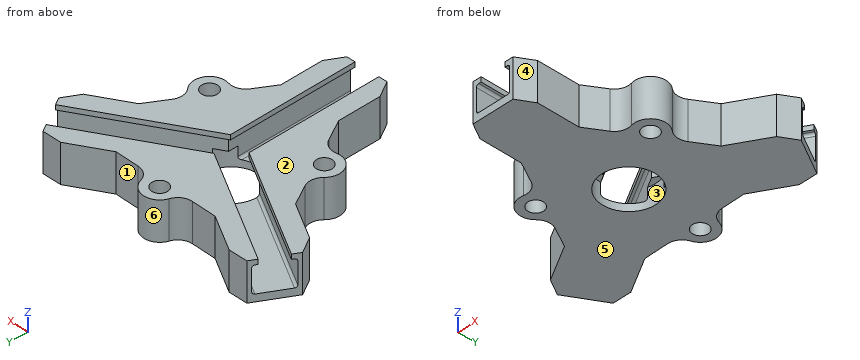
```python
from build123d import *

# Parameters (mm, degrees)
SKETCH1_R                        = 1.65
SKETCH1_R_2                      = 2.565
BOSS_EXTRUDE2_DEPTH              = 8
CUT_EXTRUDE1_REACH               = 80.832
CUT_EXTRUDE1_OFFSET_FROM_SURFACE = 13
CUT_EXTRUDE2_REACH               = 61.944
CUT_EXTRUDE2_OFFSET_FROM_SURFACE = 13
CUT_EXTRUDE3_REACH               = 80.174
CUT_EXTRUDE3_OFFSET_FROM_SURFACE = 13
FILLET1_R                        = 3
FILLET2_R                        = 0.5
SKETCH5_R                        = 5.6
CUT_EXTRUDE4_DEPTH               = 4


with BuildPart() as part:
    # Sketch1 → Boss-Extrude2 (new body)
    with BuildSketch(Plane.XY):
        with BuildLine():
            Line((-15.818539514, 20.899253914), (-23.777051469, 20.899253914))
            Line((-23.777051469, 20.899253914), (-31.392628778, 25.071578724))
            Line((-31.392628778, 25.071578724), (-35.221090626, 24.985827798))
            Line((-35.221090626, 24.985827798), (-39.387147416, 17.381691254))
            Line((-39.387147416, 17.381691254), (-37.398654012, 14.109021499))
            Line((-37.398654012, 14.109021499), (-29.783076702, 9.93669669))
            Line((-29.783076702, 9.93669669), (-25.956088039, 3.258254515))
            ThreePointArc((-25.956088039, 3.258254515), (-28.308678707, -1.639592518), (-22.893505274, -2.086230066))
            Line((-22.893505274, -2.086230066), (-18.931323152, -9.000597084))
            Line((-18.931323152, -9.000597084), (-18.736873775, -17.682042904))
            Line((-18.736873775, -17.682042904), (-16.748380371, -20.954712658))
            Line((-16.748380371, -20.954712658), (-8.079976555, -20.7605554))
            Line((-8.079976555, -20.7605554), (-6.240008112, -17.402134719))
            Line((-6.240008112, -17.402134719), (-6.434457489, -8.7206889))
            Line((-6.434457489, -8.7206889), (-2.549592829, -2.09153546))
            ThreePointArc((-2.549592829, -2.09153546), (2.845157596, -1.667339925), (0.578670581, 3.246549635))
            Line((0.578670581, 3.246549635), (4.66331299, 10.216604874))
            Line((4.66331299, 10.216604874), (12.084440923, 14.725725884))
            Line((12.084440923, 14.725725884), (13.924409366, 18.084146564))
            Line((13.924409366, 18.084146564), (9.42206234, 25.49412585))
            Line((9.42206234, 25.49412585), (5.593600493, 25.408374924))
            Line((5.593600493, 25.408374924), (-1.82752744, 20.899253914))
            Line((-1.82752744, 20.899253914), (-9.628901603, 20.899253914))
            ThreePointArc((-9.628901603, 20.899253914), (-12.723720558, 25.335848494), (-15.818539514, 20.899253914))
        make_face()
        Circle(SKETCH1_R, mode=Mode.SUBTRACT)
        with Locations((-25.447441117, 0)):
            Circle(SKETCH1_R, mode=Mode.SUBTRACT)
        with Locations((-12.723720558, 22.038130468)):
            Circle(SKETCH1_R, mode=Mode.SUBTRACT)
        with Locations((-12.723720558, 7.346043489)):
            Circle(SKETCH1_R_2, mode=Mode.SUBTRACT)
    extrude(amount=BOSS_EXTRUDE2_DEPTH)

    # Cut-Extrude1: up to this face of the body (flat: up to its plane, moved by the offset)
    cut_extrude1_end = Plane(part.part.faces().sort_by_distance((-27.869582371, 6.597475602, 4))[0]).offset(-CUT_EXTRUDE1_OFFSET_FROM_SURFACE)
    # Sketch2 → Cut-Extrude1 (cut, up to the picked face)
    with BuildSketch(Plane(origin=(18.195090402, 11.055444017, 0), x_dir=(0, 0, -1), z_dir=(0.854611923, 0.519267234, 0)), mode=Mode.PRIVATE) as cut_extrude1_sk1:
        Polygon((-1.5, 8.974437732), (-1.5, 16.145015669), (-7, 16.145015669), (-7, 15.145015669), (-8, 15.145015669), (-8, 9.974437732), (-7, 9.974437732), (-7, 8.974437732), align=None)
    cut_extrude1_tool1 = split(extrude(cut_extrude1_sk1.sketch, amount=-CUT_EXTRUDE1_REACH, mode=Mode.PRIVATE), bisect_by=cut_extrude1_end, keep=Keep.BOTH, mode=Mode.PRIVATE)
    add(cut_extrude1_tool1.solids().sort_by_distance((11.673236, 21.789136, 4.626706))[0], mode=Mode.SUBTRACT)

    # Cut-Extrude2: up to this face of the body (flat: up to its plane, moved by the offset)
    cut_extrude2_end = Plane(part.part.faces().sort_by_distance((-5.728214521, 20.899253914, 4))[0]).offset(-CUT_EXTRUDE2_OFFSET_FROM_SURFACE)
    # Sketch3 → Cut-Extrude2 (cut, up to the picked face)
    with BuildSketch(Plane(origin=(0.460715831, -20.569258657, 0), x_dir=(0.999749253, 0.022392655, 0), z_dir=(0.022392655, -0.999749253, 0)), mode=Mode.PRIVATE) as cut_extrude2_sk1:
        Polygon((-16.463412412, 1.5), (-9.292834476, 1.5), (-9.292834476, 7), (-10.292834476, 7), (-10.292834476, 8), (-15.463412412, 8), (-15.463412412, 7), (-16.463412412, 7), align=None)
    cut_extrude2_tool1 = split(extrude(cut_extrude2_sk1.sketch, amount=-CUT_EXTRUDE2_REACH, mode=Mode.PRIVATE), bisect_by=cut_extrude2_end, keep=Keep.BOTH, mode=Mode.PRIVATE)
    add(cut_extrude2_tool1.solids().sort_by_distance((-12.414178, -20.857634, 4.626706))[0], mode=Mode.SUBTRACT)

    # Cut-Extrude3: up to this face of the body (flat: up to its plane, moved by the offset)
    cut_extrude3_end = Plane(part.part.faces().sort_by_distance((2.620991785, 6.731577255, 4))[0]).offset(-CUT_EXTRUDE3_OFFSET_FROM_SURFACE)
    # Sketch4 → Cut-Extrude3 (cut, up to the picked face)
    with BuildSketch(Plane(origin=(-37.618496326, 20.609939227, 0), x_dir=(0, 0, 1), z_dir=(-0.877004578, 0.480482019, 0)), mode=Mode.PRIVATE) as cut_extrude3_sk1:
        Polygon((1.5, 4.23958464), (1.5, -2.930993297), (7, -2.930993297), (7, -1.930993297), (8, -1.930993297), (8, 3.23958464), (7, 3.23958464), (7, 4.23958464), align=None)
    cut_extrude3_tool1 = split(extrude(cut_extrude3_sk1.sketch, amount=-CUT_EXTRUDE3_REACH, mode=Mode.PRIVATE), bisect_by=cut_extrude3_end, keep=Keep.BOTH, mode=Mode.PRIVATE)
    add(cut_extrude3_tool1.solids().sort_by_distance((-37.304119, 21.18376, 4.626706))[0], mode=Mode.SUBTRACT)

    # Fillet1
    fillet1_edges = [part.edges().sort_by_distance(p)[0] for p in [
        (-2.549592829, -2.09153546, 4),
        (-22.893505274, -2.086230066, 4),
        (-25.956088039, 3.258254515, 4),
        (-15.818539514, 20.899253914, 4),
        (-9.628901603, 20.899253914, 4),
        (0.578670581, 3.246549635, 4),
    ]]
    fillet(fillet1_edges, radius=FILLET1_R)

    # Fillet2
    fillet2_edges = [part.edges().sort_by_distance(p)[0] for p in [
        (2.066272904, 11.756664371, 1.5),
        (2.066272904, 11.756664371, 7),
        (-9.116100814, -7.994563327, 7),
        (-9.116100814, -7.994563327, 1.5),
        (-16.297456112, -7.593688192, 7),
        (-16.297456112, -7.593688192, 1.5),
        (-1.177236693, 18.176338061, 1.5),
        (-1.177236693, 18.176338061, 7),
        (-23.873719146, 17.913791789, 7),
        (-23.873719146, 17.913791789, 1.5),
        (-27.811564847, 11.894993235, 7),
        (-27.811564847, 11.894993235, 1.5),
    ]]
    fillet(fillet2_edges, radius=FILLET2_R)

    # Sketch5 → Cut-Extrude4 (cut)
    with BuildSketch(Plane(origin=(0, 0, 0), x_dir=(-1, 0, 0), z_dir=(0, 0, -1))):
        with Locations((12.723720558, 7.346043489)):
            Circle(SKETCH5_R)
    extrude(amount=-CUT_EXTRUDE4_DEPTH, mode=Mode.SUBTRACT)


solid = part.part
```
Check sheet for the modelled part. Datum: model origin and axes. Units: mm. Face numbers are marked on the shaded views. A direction names the side the tool comes from. Round coordinates to 2 decimals unless told otherwise and drop trailing zeros. Answer as CSV lines item,"result". Start each with the question number.
1) Section check A-A (y = -1). Give the number of separate pieces and of enclosed holes in the cut face, then the cut area to 3 significant figures.
2) Scan lines: probe 1 along X at (y, z) = (-1, 5.75) (3 decimals); probe 2 along X at (y, z) = (16.5, 2); probe 3 along Z at (x, y) = (-28.5, 18). Record each from-to range of solid material in increasing order.
3) Tool access check on the marked faces 1, 2 and 3. Record the directions out of +Z, -Z, +X, -X, +Y, -Y that give a thin tool (end or side, any length) a straight path to the whole face; none if there is none.
4) Draft check along X on the marked faces 4, 5 and 6. Enter one of: +X half, -X half, draft (parallel to the pull), parting line (faces both ways), or undercut.
5) Depth check by flat-ended pin: pin 1 (5.5 mm diameter, centred on x = 5, y = 17.5, fed in from +Z); pin 2 (2.5 mm diameter, centred on x = -21.5, z = 3.5, fed in from +Y); pin 3 (2 mm diameter, centred on x = 1, z = 1, fed in from -Y); pin 4 (3 mm diameter, centred on y = 2.5, z = 1.5, fed in from -X). Enter the tip coordinate at first touch or a pass-through.
Determined:
1,separate pieces,"3"
1,enclosed holes,"0"
1,area,"167 mm^2"
2,probe 1,"-28.59 to -26.76, -24.135 to -16.445, -9.273 to -1.312, 1.312 to 3.142"
2,probe 2,"-38.85 to -36.22, -21.29 to -3.94, 9.87 to 13.06"
2,probe 3,"0 to 1.5"
3,face 1,"+Z, -Z, +Y"
3,face 2,"+Z, +X, -X, +Y, -Y"
3,face 3,"-Z"
4,face 4,"+X half"
4,face 5,"draft"
4,face 6,"undercut"
5,pin 1,"z = 8"
5,pin 2,"y = 20.9"
5,pin 3,"y = -3.3"
5,pin 4,"x = -28.59"
